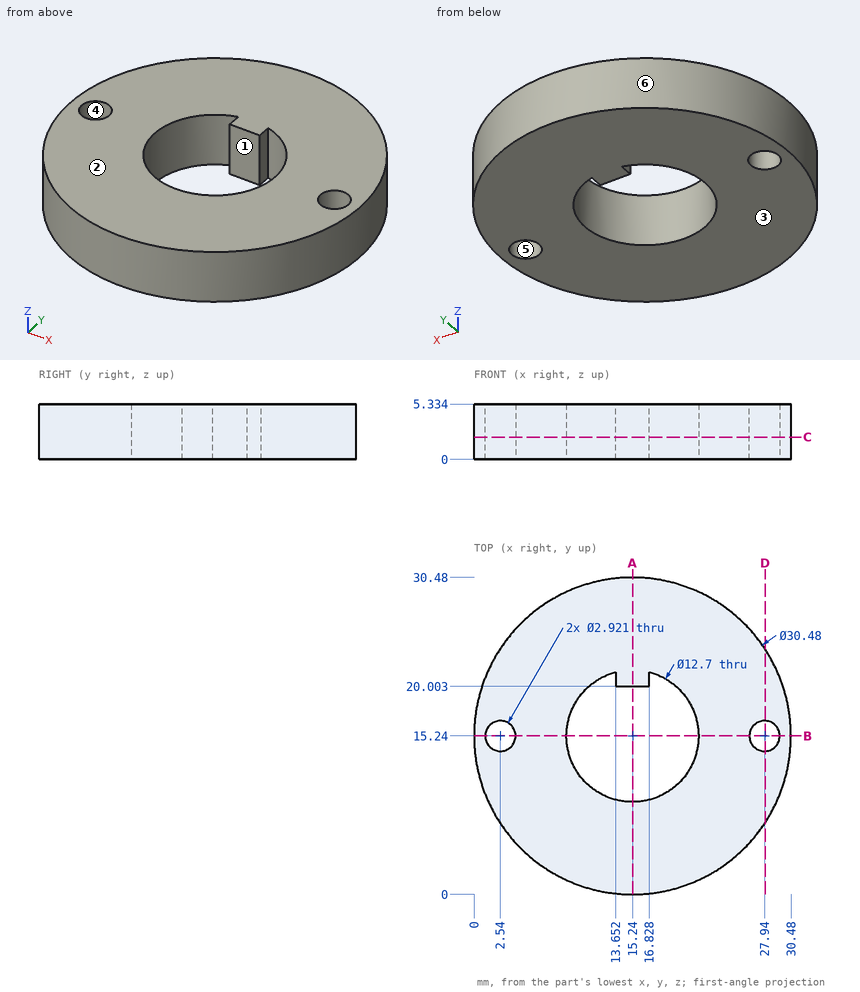
Print and shaded views of the part. All mm, measured from the part's lowest x, y and z. A direction names the side the tool comes from. Give positions to 0.01 mm unless a question says otherwise; leave off trailing zeros. Write each loop counter-clockwise with the first axis right and the second up, starting at its lowest first coordinate (ties: lowest second). Pieces come first, ordered by that corner, then holes. Notation, with made-up numbers: (42.5, 80) - (60.5, 80) arc R17 cw to (60.5, 93) - close; hole circle Ø9 at (10.5, 75.25). An arc over 180 degrees is marked (long way). One line per question, with ' | ' between items. Start each with the question number.
(1) Slice it at C-C on z = 2.15. Write the cut outline in (x, y).
(2) 3-axis set-ups, long thin cutter, end or side, ignore diameter. For the marked faces 1 and 2: which of +Z, -Z, +X, -X, +Y, -Y reach the whole face in a straight line?
(3) Slice it at D-D on x = 28. Write the cut outline in (y, z) (1 decimal).
(4) Two-plate mould, pull along X, no slides. Class the marked faces 3, 4, 5 and 6: +X half, -X half, draft (parallel to the pull), parting line (faces both ways), or undercut.
(5) Pin check, flat tips, straight feed: P1, Ø1.5, axis at y = 21, z = 2.5, coming from the -X side; P2, Ø3, axis at y = 26.5, z = 4.5, coming from the +X side (1 decimal); P3, Ø3, axis at y = 4.5, z = 1.5, coming from the +X side. Stop position of each tip, or through.
(6) Slice it at A-A on x = 15.24. Write the cut outline in (y, z) (1 decimal), plus the area to 3 significant figures.
(7) Slice it at B-B on y = 15.24. Write the cut outline in (x, z) (1 decimal).
(8) Wall check: line 1 along X through (y, z) = (15, 0.65) (1 decimal); line 2 along X through (y, z) = (19, 3.3) (1 decimal). Give the ranges that are in metal, low to high. Write a range as from..to.
Results below:
1) outline: circle Ø30.48 at (15.24, 15.24); hole circle Ø2.92 at (2.54, 15.24); hole (13.65, 20) - (13.65, 21.39) arc R6.35 ccw (long way) to (16.83, 21.39) - (16.83, 20) - close; hole circle Ø2.92 at (27.94, 15.24)
2) face 1: +Z, -Z | face 2: +Z, +X, -X, +Y, -Y
3) outline: (6.9, 0) - (13.8, 0) - (13.8, 5.3) - (6.9, 5.3) - close; (16.7, 0) - (23.6, 0) - (23.6, 5.3) - (16.7, 5.3) - close
4) face 3: draft | face 4: undercut | face 5: undercut | face 6: parting line
5) P1: x = 0.85 | P2: x = 26.9 | P3: x = 27.36
6) outline: (0, 0) - (8.9, 0) - (8.9, 5.3) - (0, 5.3) - close; (20, 0) - (30.5, 0) - (30.5, 5.3) - (20, 5.3) - close | area: 103 mm^2
7) outline: (0, 0) - (1.1, 0) - (1.1, 5.3) - (0, 5.3) - close; (4, 0) - (8.9, 0) - (8.9, 5.3) - (4, 5.3) - close; (21.6, 0) - (26.5, 0) - (26.5, 5.3) - (21.6, 5.3) - close; (29.4, 0) - (30.5, 0) - (30.5, 5.3) - (29.4, 5.3) - close
8) line 1: 0..1.1, 4..8.9, 21.6..26.5, 29.4..30.5 | line 2: 0.5..10.1, 20.4..30
